from build123d import *

# Parameters (mm, degrees)
BOSS_EXTRUDE1_DEPTH      = 7.5
BOSS_EXTRUDE1_DEPTH_BACK = 7.5
CUT_EXTRUDE3_REACH       = 31.568
SKETCH5_R                = 1.5
BOSS_EXTRUDE2_DEPTH      = 3.7
BOSS_EXTRUDE2_DEPTH_BACK = 3.7
SKETCH6_R                = 1.2
FILLET1_R                = 8
FILLET2_R                = 5
CUT_EXTRUDE4_START       = -12.346261552
CUT_EXTRUDE4_OUTLINE_R   = 0.5
CUT_EXTRUDE4_DEPTH       = 22.047733515


# Read off the part's stored shape, not the designer's step: Cut-Extrude4
with BuildPart() as part:
    # Sketch1 → Boss-Extrude1 (new, two sides: drawn at the far end of the back side and taken through both)
    with BuildSketch(Plane(origin=(0, 0, 0), x_dir=(-1, 0, 0), z_dir=(0, 1, 0)).offset(-BOSS_EXTRUDE1_DEPTH_BACK)):
        with BuildLine():
            Line((-13.8, -7.5), (13.8, -7.5))
            Line((13.8, -7.5), (13.8, 7.5))
            Line((13.8, 7.5), (-6.3, 7.5))
            Line((-6.3, 7.5), (-12.102943725, 1.697056275))
            ThreePointArc((-12.102943725, 1.697056275), (-11.582689122, -0.918440238), (-13.8, -2.4))
            Line((-13.8, -2.4), (-13.8, -7.5))
        make_face()
    extrude(amount=BOSS_EXTRUDE1_DEPTH + BOSS_EXTRUDE1_DEPTH_BACK)

    # Sketch5 → Cut-Extrude3 (cut, up to next)
    with BuildSketch(Plane.YZ.offset(13.8), mode=Mode.PRIVATE) as cut_extrude3_sk1:
        with Locations(Location((-2.25, -4.95, 0), (0, 0, 270))):
            Circle(SKETCH5_R)
    cut_extrude3_tool1 = extrude(cut_extrude3_sk1.sketch, amount=-CUT_EXTRUDE3_REACH, mode=Mode.PRIVATE) & part.part
    # Sketch5 → Cut-Extrude3 (cut, up to next)
    with BuildSketch(Plane.YZ.offset(13.8), mode=Mode.PRIVATE) as cut_extrude3_sk2:
        with Locations(Location((2.25, -4.95, 0), (0, 0, 270))):
            Circle(SKETCH5_R)
    cut_extrude3_tool2 = extrude(cut_extrude3_sk2.sketch, amount=-CUT_EXTRUDE3_REACH, mode=Mode.PRIVATE) & part.part
    add(cut_extrude3_tool1.solids().sort_by_distance((13.8, -2.25, -4.95))[0], mode=Mode.SUBTRACT)
    add(cut_extrude3_tool2.solids().sort_by_distance((13.8, 2.25, -4.95))[0], mode=Mode.SUBTRACT)

    # Sketch6 → Boss-Extrude2 (add, two sides: drawn at the far end of the back side and taken through both)
    with BuildSketch(Plane(origin=(0, 0, 0), x_dir=(-1, 0, 0), z_dir=(0, 1, 0)).offset(-BOSS_EXTRUDE2_DEPTH_BACK)):
        with BuildLine():
            Line((-12.102943725, 1.697056275), (-12.244365081, 1.555634919))
            ThreePointArc((-12.244365081, 1.555634919), (-15.832534972, 0.841903551), (-13.8, -2.2))
            Line((-13.8, -2.2), (-13.8, -2.4))
            ThreePointArc((-13.8, -2.4), (-11.582689122, -0.918440238), (-12.102943725, 1.697056275))
        make_face()
        with Locations(Location((-13.8, 0, 0), (0, 0, 90))):
            Circle(SKETCH6_R, mode=Mode.SUBTRACT)
    extrude(amount=BOSS_EXTRUDE2_DEPTH + BOSS_EXTRUDE2_DEPTH_BACK)

    # Fillet1
    fillet1_edges = [part.edges().sort_by_distance(p)[0] for p in [
        (-13.8, 0, 7.5),
    ]]
    fillet(fillet1_edges, radius=FILLET1_R)

    # Fillet2
    # the kernel refuses this fillet: 5 mm, written as the material it takes off along each edge
    with BuildSketch(Plane(origin=(26.3, -7.5, -7.5), x_dir=(0, 1, 0), z_dir=(-1, 0, 0)), Plane(origin=(26.3, 7.5, -7.5), x_dir=(0, 0, 1), z_dir=(-1, 0, 0))) as fillet2_piece_1:
        with BuildLine():
            CenterArc((FILLET2_R, -FILLET2_R), FILLET2_R, 90, 90)
            Line((0, -FILLET2_R), (0, 0))
            Line((0, 0), (FILLET2_R, 0))
        make_face()
    extrude(amount=52.6, mode=Mode.SUBTRACT)
    with BuildSketch(Plane(origin=(-5.8, 7.5, 7.5), x_dir=(0, 0, -1), z_dir=(1, 0, 0)), Plane(origin=(-5.8, -7.5, 7.5), x_dir=(0, 1, 0), z_dir=(1, 0, 0))) as fillet2_piece_2:
        with BuildLine():
            CenterArc((FILLET2_R, -FILLET2_R), FILLET2_R, 90, 90)
            Line((0, -FILLET2_R), (0, 0))
            Line((0, 0), (FILLET2_R, 0))
        make_face()
    extrude(amount=24.6, mode=Mode.SUBTRACT)
    with BuildSketch(Plane(origin=(-13.8, 7.5, -20), x_dir=(1, 0, 0), z_dir=(0, 0, 1)), Plane(origin=(-13.8, -7.5, -20), x_dir=(0, 1, 0), z_dir=(0, 0, 1))) as fillet2_piece_3:
        with BuildLine():
            CenterArc((FILLET2_R, -FILLET2_R), FILLET2_R, 90, 90)
            Line((0, -FILLET2_R), (0, 0))
            Line((0, 0), (FILLET2_R, 0))
        make_face()
    extrude(amount=19.5, mode=Mode.SUBTRACT)
    with BuildSketch(Plane(origin=(-5.8, 7.5, -0.5), x_dir=(0, 0, 1), z_dir=(1, 0, 0))) as fillet2_piece_4:
        with BuildLine():
            CenterArc((8 - FILLET2_R, FILLET2_R), FILLET2_R, 270, 90)
            Line((8, FILLET2_R), (8, 0))
            Line((8, 0), (8 - FILLET2_R, 0))
        make_face()
    revolve(axis=Axis((-5.8, 7.5, -0.5), (0, -1, 0)), revolution_arc=90, mode=Mode.SUBTRACT)
    with BuildSketch(Plane(origin=(-5.8, -7.5, -0.5), x_dir=(0, 0, 1), z_dir=(1, 0, 0))) as fillet2_piece_5:
        with BuildLine():
            CenterArc((8 - FILLET2_R, -FILLET2_R), FILLET2_R, 0, 90)
            Line((8 - FILLET2_R, 0), (8, 0))
            Line((8, 0), (8, -FILLET2_R))
        make_face()
    revolve(axis=Axis((-5.8, -7.5, -0.5), (0, -1, 0)), revolution_arc=90, mode=Mode.SUBTRACT)

    # Cut-Extrude4 outline → Cut-Extrude4 (cut)
    with BuildSketch(Plane.YZ.offset(CUT_EXTRUDE4_START)):
        with Locations((0, 4.598528137)):
            Circle(CUT_EXTRUDE4_OUTLINE_R)
    extrude(amount=CUT_EXTRUDE4_DEPTH, mode=Mode.SUBTRACT)


solid = part.part
The listing builds one solid part. Answer for the finished solid, in the listing's coordinates (mm). A direction names the side the tool comes from. Coordinates: 2 decimals unless noted, no trailing zeros. Write each loop counter-clockwise with the first axis right and the second up, starting at its lowest first coordinate (ties: lowest second). Pieces come first, ordered by that corner, then holes. Notation, with made-up numbers: M -39.75,-21 L -4.75,-21 A22 ccw -4.75,-4 Z; hole C 54.25,17.5 d11. An arc over 180 degrees is marked long. Use one line per item in the form item = value.
Item 1: The mould has two halves that part along Y. Classify faces 1 (the face through (0.193, 0.786, -4.625)), 2 (the face through (11.568, 5.573, -0.882)), 3 (the face through (3, -7.5, 0)): released by +Y, released by -Y, zero draft, split by the parting line, or undercut.
Model answer:
face_1 = undercut
face_2 = zero draft
face_3 = released by -Y
Item 2: Find the intervals of material crossed by probe 1 along Z at (x, y) = (4.5, 2.25); probe 2 along Y at (x, z) = (-7, -4); probe 3 along Y at (x, z) = (4, -6), in increasing order.
Model answer:
probe_1 = -7.5 to -6.45, -3.45 to 7.5
probe_2 = -7.27 to -3.41, -1.09 to 1.09, 3.41 to 7.27
probe_3 = -6.07 to -3.32, -1.18 to 1.18, 3.32 to 6.07
Item 3: For faces 4 (the face through (11.568, -5.627, -0.882)), 5 (the face through (13.8, 0, -4)), 6 (the face through (0, 0, 7.5)), determine the directions among +Z, -Z, +X, -X, +Y, -Y from which every point of the face is accessible in a straight line to the end or side of a thin tool.
Model answer:
face_4 = +X, -Y
face_5 = -Z, +X, +Y, -Y
face_6 = +Z, +X, -X, +Y, -Y
Item 4: Find section A-A, the plane x = 6.75. Give the vertices of the cut face in (y, z), plus the area to 3 significant figures.
Model answer:
outline = M -7.5,-2.5 A5 ccw -2.5,-7.5 L 2.5,-7.5 A5 ccw 7.5,-2.5 L 7.5,2.5 A5 ccw 4.57,7.05 L -4.57,7.05 A5 ccw -7.5,2.5 Z; hole C -2.25,-4.95 d3; hole C 0,4.6 d1; hole C 2.25,-4.95 d3
area = 185 mm2
Item 5: Find section C-C, the plane x = 10.5. Give the vertices of the cut face in (y, z), plus the area to 3 significant figures.
Model answer:
outline = M -7.5,-2.5 A5 ccw -2.5,-7.5 L 2.5,-7.5 A5 ccw 7.5,-2.5 L 7.5,2.5 A5 ccw 7.44,3.3 L -7.44,3.3 A5 ccw -7.5,2.5 Z; hole C -2.25,-4.95 d3; hole C 2.25,-4.95 d3
area = 137 mm2
Item 6: Find section D-D, the plane z = -3. Give the vertices of the cut face in (x, y), plus the area to 3 significant figures.
Model answer:
outline = M -13.8,-2.5 A5 ccw -9.3,-7.47 L 13.8,-7.47 L 13.8,7.47 L -9.3,7.47 A5 ccw -13.8,2.5 Z
area = 402 mm2
Item 7: Given P1, Ø2, axis at x = 6, y = 5, coming from the +Z side; P2, Ø1.6, axis at y = 2.5, z = -4.5, coming from the +X side; P3, Ø6, axis at y = 5, z = -3, coming from the +X side; P4, Ø1.5, axis at y = 6, z = 0.5, coming from the +X side, each flat-ended and moving along its own axis, determine where each tip first touches the part or whether it passes through.
Model answer:
P1 = 7.27
P2 = through
P3 = 15.98
P4 = 11.75
Item 8: Find section B-B, the plane z = -4.95. Give the vertices of the cut face in (x, y), plus the area to 3 significant figures.
Model answer:
outline = M -13.8,-0.75 L 13.8,-0.75 L 13.8,0.75 L -13.8,0.75 Z; M -13.64,-3.75 A5 ccw -11.25,-6.86 L 13.8,-6.86 L 13.8,-3.75 Z; M -13.64,3.75 L 13.8,3.75 L 13.8,6.86 L -11.25,6.86 A5 ccw Z
area = 207 mm2
